from build123d import *

# Parameters (mm, degrees)
SKETCH1_W           = 203.2
SKETCH1_H           = 165.1
SKETCH1_R           = 1.5875
SKETCH1_W_2         = 22.0345
SKETCH1_H_2         = 18.7325
BOSS_EXTRUDE1_DEPTH = 6.35


with BuildPart() as part:
    # Sketch1 → Boss-Extrude1 (new body)
    with BuildSketch(Plane.XY):
        with Locations((-29.151775306, -7.158362635)):
            Rectangle(SKETCH1_W, SKETCH1_H)
        with Locations((66.098224694, 37.291637365)):
            Circle(SKETCH1_R, mode=Mode.SUBTRACT)
        with Locations((66.098224694, -51.608362635)):
            Circle(SKETCH1_R, mode=Mode.SUBTRACT)
        with Locations((58.128974694, 62.723387365)):
            Rectangle(SKETCH1_W_2, SKETCH1_H_2, mode=Mode.SUBTRACT)
        with Locations((-116.432525306, 62.723387365)):
            Rectangle(SKETCH1_W_2, SKETCH1_H_2, mode=Mode.SUBTRACT)
        with Locations((58.128974694, -77.040112635)):
            Rectangle(SKETCH1_W_2, SKETCH1_H_2, mode=Mode.SUBTRACT)
        with Locations((-116.432525306, -77.040112635)):
            Rectangle(SKETCH1_W_2, SKETCH1_H_2, mode=Mode.SUBTRACT)
    extrude(amount=BOSS_EXTRUDE1_DEPTH)


solid = part.part
Design review of the part built by this model. Coordinates are the model's own, in mm. A direction names the side the tool comes from. Give positions to 0.01 mm unless a question says otherwise; leave off trailing zeros. Order: outer loops, then holes, each group sorted by start corner. A loop starts at its lowest first (then second) coordinate and runs counter-clockwise, first axis right, second up. Notation, with made-up numbers: (76, -35) - (87, -35) arc R16 ccw to (87, -29) - close; hole circle Ø8 at (49, -37.5). An arc over 180 degrees is marked (long way). Write item = value, one per line. Start each with the question number.
Q1. We need section A-A on z = 5. State the section outline as (x, y) points (1 decimal), plus the area to 3 significant figures.
Q2. Tool access review of faces 1 (the face through (58, -86.406, 3)), 2 (the face through (-31, -89.708, 3)): name each direction out of +Z, -Z, +X, -X, +Y, -Y from which nothing blocks a thin tool from reaching the whole face with its end or side.
Q3. Mouldability with a two-part tool opening along X and no side actions: class faces 3 (the face through (-31, -6, 0)), 4 (the face through (-130.752, -8, 3)), 5 (the face through (-105.415, -77, 3)) as released by +X, released by -X, zero draft, split by the parting line, or undercut.
Q4. To check wall thickness, follow L1, parallel to Y at x = -109.5, z = 1.75; L2, parallel to X at y = 61.5, z = 2.25; L3, parallel to X at y = 36, z = 4.5. State the ranges of each line that lie inside material, in increasing order. Write a range as from..to.
Working result:
q1.outline = (-130.8, -89.7) - (72.4, -89.7) - (72.4, 75.4) - (-130.8, 75.4) - close; hole (-127.4, -86.4) - (-105.4, -86.4) - (-105.4, -67.7) - (-127.4, -67.7) - close; hole (-127.4, 53.4) - (-105.4, 53.4) - (-105.4, 72.1) - (-127.4, 72.1) - close; hole (47.1, -86.4) - (69.1, -86.4) - (69.1, -67.7) - (47.1, -67.7) - close; hole (47.1, 53.4) - (69.1, 53.4) - (69.1, 72.1) - (47.1, 72.1) - close; hole circle Ø3.2 at (66.1, -51.6); hole circle Ø3.2 at (66.1, 37.3)
q1.area = 31,900 mm²
q2.face_1 = +Z, -Z
q2.face_2 = +Z, -Z, +X, -X, -Y
q3.face_3 = zero draft
q3.face_4 = released by -X
q3.face_5 = undercut
q4.L1 = -89.71..-86.41, -67.67..53.36, 72.09..75.39
q4.L2 = -130.75..-127.45, -105.42..47.11, 69.15..72.45
q4.L3 = -130.75..65.18, 67.02..72.45
